Input: dimensioned drawing with shaded views. Units: mm. Origin: part minimum x, y, z. Round coordinates to 2 decimals unless told otherwise and drop trailing zeros. Order: outer loops, then holes, each group sorted by start corner. A loop starts at its lowest first (then second) coordinate and runs counter-clockwise, first axis right, second up.
Item 1: Cut plane A-A on z = 1.7. Output: boundary loops of the cut face in (x, y).
Item 2: Cut plane B-B on x = 9.25. Output: boundary loops of the cut face in (y, z).
Item 3: Mould query, pull axis Y, two halves, no side actions, for the marked faces 1, 2, 3 and 4. Classes: released by +Y, released by -Y, zero draft, split by the parting line, or undercut.
Item 4: Line query: L1, parallel to X at y = 4, z = 1 (1 decimal); L2, parallel to X at y = 5.25, z = 0.65; L3, parallel to Y at x = 4.75, z = 3. Output: solid intervals per line, ascending.
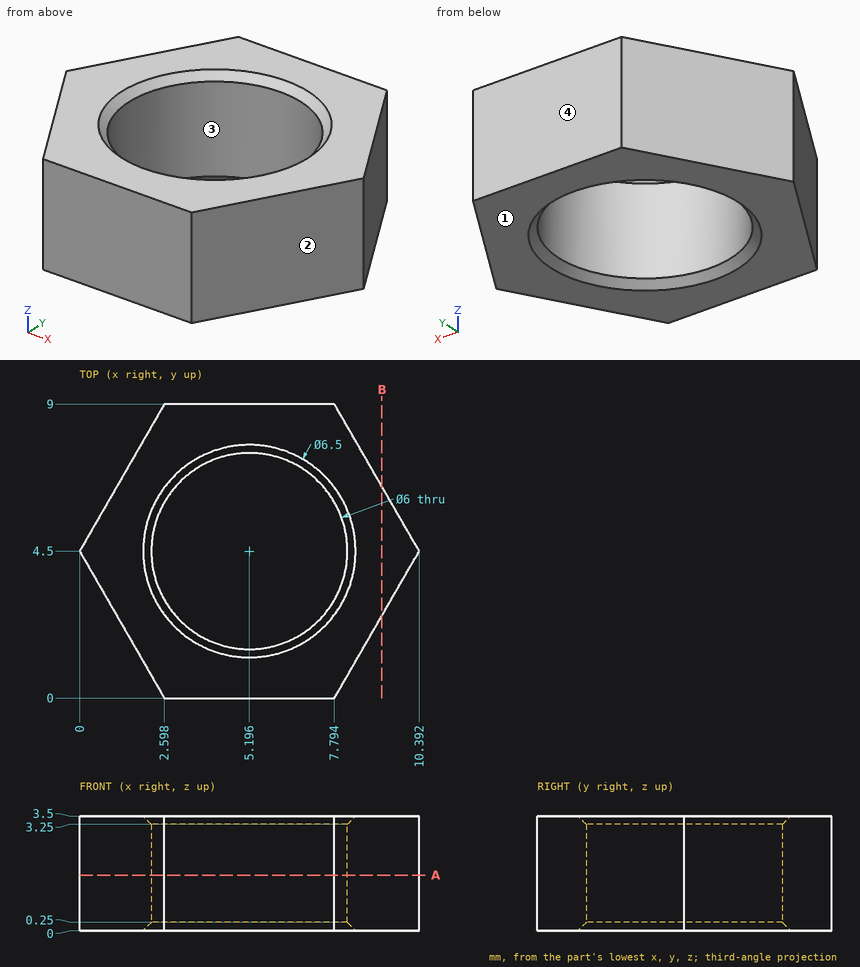
From the geometry:
1. outline: (0, 4.5) - (2.6, 0) - (7.79, 0) - (10.39, 4.5) - (7.79, 9) - (2.6, 9) - close; hole circle Ø6 at (5.2, 4.5)
2. outline: (2.52, 0) - (6.48, 0) - (6.48, 3.5) - (2.52, 3.5) - close
3. face 1: zero draft
3. face 2: released by -Y
3. face 3: undercut
3. face 4: released by +Y
4. L1: x = 0.3 to 2.2, 8.2 to 10.1
4. L2: x = 0.43 to 2.29, 8.1 to 9.96
4. L3: y = 0 to 1.53, 7.47 to 9
